For this review, take the finished solid that the model builds, in its own axes (mm). Face numbers are marked on the shaded views. Coordinates: 2 decimals unless noted, no trailing zeros. Write each loop counter-clockwise with the first axis right and the second up, starting at its lowest first coordinate (ties: lowest second). Pieces come first, ordered by that corner, then holes.
```python
from build123d import *

# Parameters (mm, degrees)
SKETCH_1_W          = 200
SKETCH_1_H          = 100
EXTRUDE_1_DEPTH     = 15
SKETCH_2_R          = 35
EXTRUDE_2_DEPTH     = 20
SKETCH_3_R          = 25
CUT_EXTRUDE_1_DEPTH = 227.329405955
SKETCH_4_R          = 10
CUT_EXTRUDE_2_DEPTH = 225.499443206
FILLET_1_R          = 10


with BuildPart() as part:
    # Эскиз1 → Бобышка-Вытянуть1 (new body)
    with BuildSketch(Plane(origin=(0, 0, 0), x_dir=(1, 0, 0), z_dir=(0, 1, 0))):
        with Locations((100, 50)):
            Rectangle(SKETCH_1_W, SKETCH_1_H)
    extrude(amount=EXTRUDE_1_DEPTH)

    # Эскиз2 → Бобышка-Вытянуть2 (add)
    with BuildSketch(Plane(origin=(0, 15, 0), x_dir=(1, 0, 0), z_dir=(0, 1, 0))):
        with Locations(Location((100, 50, 0), (0, 0, 270))):
            Circle(SKETCH_2_R)
    extrude(amount=EXTRUDE_2_DEPTH)

    # Эскиз3 → Вырез-Вытянуть1 (cut, through all)
    with BuildSketch(Plane(origin=(0, 35, 0), x_dir=(1, 0, 0), z_dir=(0, 1, 0))):
        with Locations(Location((100, 50, 0), (0, 0, 270))):
            Circle(SKETCH_3_R)
    extrude(amount=-CUT_EXTRUDE_1_DEPTH, mode=Mode.SUBTRACT)

    # Эскиз4 → Вырез-Вытянуть2 (cut, through all)
    with BuildSketch(Plane(origin=(0, 15, 0), x_dir=(1, 0, 0), z_dir=(0, 1, 0))):
        with Locations(Location((20, 20, 0), (0, 0, 270))):
            Circle(SKETCH_4_R)
        with Locations(Location((20, 80, 0), (0, 0, 270))):
            Circle(SKETCH_4_R)
        with Locations(Location((180, 80, 0), (0, 0, 270))):
            Circle(SKETCH_4_R)
        with Locations(Location((180, 20, 0), (0, 0, 270))):
            Circle(SKETCH_4_R)
    extrude(amount=-CUT_EXTRUDE_2_DEPTH, mode=Mode.SUBTRACT)

    # Скругление1
    fillet_1_edges = [part.edges().sort_by_distance(p)[0] for p in [
        (0, 7.5, 0),
        (0, 7.5, -100),
        (200, 7.5, -100),
        (200, 7.5, 0),
    ]]
    fillet(fillet_1_edges, radius=FILLET_1_R)


solid = part.part
```
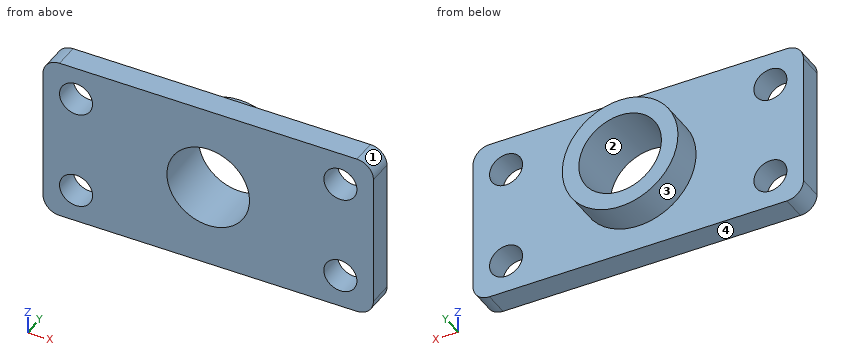
Q1. Draft analysis for pull direction X (two halves, no side actions). For the marked faces 1, 2, 3 and 4, state which applies: +X half, -X half, draft (parallel to the pull), parting line (faces both ways), or undercut.
Ans:
face 1: +X half
face 2: undercut
face 3: parting line
face 4: draft
Q2. Clearance check with flat-ended pins moving along their axes: pin 1 Ø10 at (x, z) = (111.5, -36.5) entering from -Y; pin 2 Ø10 at (x, z) = (56, -50) entering from +Y; pin 3 Ø4 at (x, y) = (80, 29) entering from +Z; pin 4 Ø12 at (x, y) = (77, 30) entering from -Z. State where each tip first meets the part, or that it passes through.
Ans:
pin 1: passes through
pin 2: stops at y = 15
pin 3: stops at z = -19.98
pin 4: stops at z = -80.59
Q3. Add section C-C (x = 180). State the section outline as (y, z) points, then the cut area to 3 significant figures.
Ans:
outline: (0, -100) - (15, -100) - (15, -90) - (0, -90) - close; (0, -70) - (15, -70) - (15, -30) - (0, -30) - close; (0, -10) - (15, -10) - (15, 0) - (0, 0) - close
area: 900 mm2
Q4. Add section B-B (z = -50). State the section outline as (x, y) points.
Ans:
outline: (0, 0) - (75, 0) - (75, 35) - (65, 35) - (65, 15) - (0, 15) - close; (125, 0) - (200, 0) - (200, 15) - (135, 15) - (135, 35) - (125, 35) - close
Q5. For probe 1 along X at (y, z) = (5, -20); probe 2 along X at (y, z) = (6.5, -11); probe 3 along Y at (x, z) = (188, -94), list the stretches that pass through material, from the lowest coordinate up.
Ans:
probe 1: x = 0 to 10, 30 to 170, 190 to 200
probe 2: x = 0 to 15.64, 24.36 to 175.64, 184.36 to 200
probe 3: y = 0 to 15
Q6. Add section D-D (y = 13). State the section outline as (x, z) points.
Ans:
outline: (0, -90) arc R10 ccw to (10, -100) - (190, -100) arc R10 ccw to (200, -90) - (200, -10) arc R10 ccw to (190, 0) - (10, 0) arc R10 ccw to (0, -10) - close; hole circle Ø20 at (20, -80); hole circle Ø20 at (20, -20); hole circle Ø50 at (100, -50); hole circle Ø20 at (180, -80); hole circle Ø20 at (180, -20)
Q7. Add section A-A (x = 100). State the section outline as (y, z) points, then the cut area to 3 significant figures.
Ans:
outline: (0, -100) - (15, -100) - (15, -85) - (35, -85) - (35, -75) - (0, -75) - close; (0, -25) - (35, -25) - (35, -15) - (15, -15) - (15, 0) - (0, 0) - close
area: 1,150 mm2
